For this review, take the finished solid that the model builds, in its own axes (mm). A direction names the side the tool comes from. Coordinates: 2 decimals unless noted, no trailing zeros. Loops run counter-clockwise (first coordinate to the right, second up) from the corner with the lowest first, then second, coordinate; pieces in that order, holes last.
1. Take a section at C-C, the plane x = -23. State the section outline as (y, z) points, then the cut area to 3 significant figures.
2. Machinability: for faces 4 (the face through (11, 4, -27)), 5 (the face through (8.8, 6, -13)), 6 (the face through (-37.564, 3.944, -30.454)), 7 (the face through (-26, 4, 22.486)), which of the approach directions +Z, -Z, +X, -X, +Y, -Y give a long, thin tool a straight path to every point of the face, cutting with its end or side? Answer none if there is none.
3. Clearance check with flat-ended pins moving along their axes: P1, Ø1.5, axis at y = 4, z = 2.5, coming from the +X side; P2, Ø5.5, axis at x = -10.61, z = 10.61, coming from the +Y side; P3, Ø1.8, axis at x = -10.5, z = 24.5, coming from the -Y side. State where each tip first meets the part, or that it passes through.
4. Take a section at D-D, the plane z = 3.5. State the section outline as (x, y) points.
5. To check wall thickness, follow probe 1 along Z at (x, y) = (-30, 1); probe 2 along X at (y, z) = (5.5, 12.5); probe 3 along X at (y, z) = (6, 12). State the ranges of each line that lie inside material, in increasing order.
6. Mouldability with a two-part tool opening along X and no side actions: class faces 1 (the face through (3, 4, 32.014)), 2 (the face through (-37.53, 3.94, 30.6)), 3 (the face through (8.899, 5.972, -27.372)) as pulls with the +X half, pulls with the -X half, needs draft (parallel to the pull), parting line crosses it, or undercut.
7. Take a section at A-A, the plane x = 0. State the section outline as (y, z) points, then the cut area to 3 significant figures.
8. Take a section at B-B, the plane z = -26. State the section outline as (x, y) points.
```python
from build123d import *

# Parameters (mm, degrees)
SKETCH1_R           = 9
SKETCH1_R_2         = 1.5
SKETCH1_W           = 17.49
SKETCH1_H           = 7
SKETCH1_W_2         = 18.51
BOSS_EXTRUDE1_DEPTH = 8
SKETCH2_R           = 3
CUT_EXTRUDE1_DEPTH  = 4
SKETCH5_R           = 1.5
CUT_EXTRUDE3_DEPTH  = 52.125968688
SKETCH5_3_R         = 3
SKETCH5_3_R_2       = 1.5
CUT_EXTRUDE4_DEPTH  = 4


with BuildPart() as part:
    # Sketch1 → Boss-Extrude1 (new body)
    with BuildSketch(Plane(origin=(0, 0, 0), x_dir=(1, 0, 0), z_dir=(0, 1, 0))):
        with BuildLine():
            Line((-33.922517503, 31.986083161), (38.983038853, 31.986083161))
            Line((38.983038853, 31.986083161), (39.05091296, -32.013916839))
            Line((39.05091296, -32.013916839), (-34.065012631, -32.013916839))
            ThreePointArc((-34.065012631, -32.013916839), (-37.566569007, -30.563524698), (-39.016961147, -27.061968322))
            Line((-39.016961147, -27.061968322), (-39.016961147, 26.891639518))
            ThreePointArc((-39.016961147, 26.891639518), (-37.52483315, 30.493955165), (-33.922517503, 31.986083161))
        make_face()
        with Locations(Location((0, 0, 0), (0, 0, 270))):
            Circle(SKETCH1_R, mode=Mode.SUBTRACT)
        with Locations(Location((10.606601718, 10.606601718, 0), (0, 0, 270))):
            Circle(SKETCH1_R_2, mode=Mode.SUBTRACT)
        with Locations(Location((-10.606601718, 10.606601718, 0), (0, 0, 90))):
            Circle(SKETCH1_R_2, mode=Mode.SUBTRACT)
        with Locations(Location((10.606601718, -10.606601718, 0), (0, 0, 90))):
            Circle(SKETCH1_R_2, mode=Mode.SUBTRACT)
        with Locations(Location((-10.606601718, -10.606601718, 0), (0, 0, 270))):
            Circle(SKETCH1_R_2, mode=Mode.SUBTRACT)
        with Locations((-26.271961147, 25.986083161)):
            Rectangle(SKETCH1_W, SKETCH1_H, mode=Mode.SUBTRACT)
        with Locations((26.728038853, 25.986083161)):
            Rectangle(SKETCH1_W_2, SKETCH1_H, mode=Mode.SUBTRACT)
        with Locations((26.728038853, -25.986083161)):
            Rectangle(SKETCH1_W_2, SKETCH1_H, mode=Mode.SUBTRACT)
        with Locations((-26.271961147, -25.986083161)):
            Rectangle(SKETCH1_W, SKETCH1_H, mode=Mode.SUBTRACT)
    extrude(amount=BOSS_EXTRUDE1_DEPTH)

    # Sketch2 → Cut-Extrude1 (cut)
    with BuildSketch(Plane(origin=(0, 8, 0), x_dir=(1, 0, 0), z_dir=(0, 1, 0))):
        with Locations(Location((10.606601718, 10.606601718, 0), (0, 0, 270))):
            Circle(SKETCH2_R)
        with Locations(Location((10.606601718, -10.606601718, 0), (0, 0, 270))):
            Circle(SKETCH2_R)
        with Locations(Location((-10.606601718, -10.606601718, 0), (0, 0, 270))):
            Circle(SKETCH2_R)
        with Locations(Location((-10.606601718, 10.606601718, 0), (0, 0, 270))):
            Circle(SKETCH2_R)
    extrude(amount=-CUT_EXTRUDE1_DEPTH, mode=Mode.SUBTRACT)

    # Sketch5 → Cut-Extrude3 (cut, through all)
    with BuildSketch(Plane.XZ):
        with Locations(Location((-10.52309756, 25.986083161, 0), (0, 0, 270))):
            Circle(SKETCH5_R)
        with Locations(Location((9.473038853, 25.986083161, 0), (0, 0, 270))):
            Circle(SKETCH5_R)
        with Locations(Location((9.473038853, -25.986083161, 0), (0, 0, 270))):
            Circle(SKETCH5_R)
        with Locations(Location((-10.52309756, -25.986083161, 0), (0, 0, 270))):
            Circle(SKETCH5_R)
    extrude(amount=-CUT_EXTRUDE3_DEPTH, mode=Mode.SUBTRACT)

    # Sketch5_3 → Cut-Extrude4 (cut)
    # profile 1 of 4: a face of its own
    with BuildSketch(Plane.XZ):
        with Locations(Location((-10.52309756, -25.986083161, 0), (0, 0, 270))):
            Circle(SKETCH5_3_R)
        with Locations(Location((-10.52309756, -25.986083161, 0), (0, 0, 270))):
            Circle(SKETCH5_3_R_2, mode=Mode.SUBTRACT)
    # profile 2 of 4: a face of its own
    with BuildSketch(Plane.XZ):
        with Locations(Location((9.473038853, -25.986083161, 0), (0, 0, 270))):
            Circle(SKETCH5_3_R)
        with Locations(Location((9.473038853, -25.986083161, 0), (0, 0, 270))):
            Circle(SKETCH5_3_R_2, mode=Mode.SUBTRACT)
    # profile 3 of 4: a face of its own
    with BuildSketch(Plane.XZ):
        with Locations(Location((9.473038853, 25.986083161, 0), (0, 0, 270))):
            Circle(SKETCH5_3_R)
        with Locations(Location((9.473038853, 25.986083161, 0), (0, 0, 270))):
            Circle(SKETCH5_3_R_2, mode=Mode.SUBTRACT)
    # profile 4 of 4: a face of its own
    with BuildSketch(Plane.XZ):
        with Locations(Location((-10.52309756, 25.986083161, 0), (0, 0, 270))):
            Circle(SKETCH5_3_R)
        with Locations(Location((-10.52309756, 25.986083161, 0), (0, 0, 270))):
            Circle(SKETCH5_3_R_2, mode=Mode.SUBTRACT)
    extrude(amount=-CUT_EXTRUDE4_DEPTH, mode=Mode.SUBTRACT)


solid = part.part
```
Results list:
1. outline: (0, -31.99) - (8, -31.99) - (8, -29.49) - (0, -29.49) - close; (0, -22.49) - (8, -22.49) - (8, 22.49) - (0, 22.49) - close; (0, 29.49) - (8, 29.49) - (8, 32.01) - (0, 32.01) - close
1. area: 400 mm2
2. face 4: -Y
2. face 5: +Y
2. face 6: -Z, -X, +Y, -Y
2. face 7: +Y, -Y
3. P1: stops at x = 39.02
3. P2: stops at y = 4
3. P3: stops at y = 4
4. outline: (-39.02, 0) - (-8.29, 0) - (-8.29, 8) - (-39.02, 8) - close; (8.29, 0) - (39.02, 0) - (39.02, 8) - (8.29, 8) - close
5. probe 1: z = -31.99 to -29.49, -22.49 to 22.49, 29.49 to 32.01
5. probe 2: x = -39.02 to -12.93, -8.28 to 8.28, 12.93 to 39.03
5. probe 3: x = -39.02 to -13.26, -7.95 to 7.95, 13.26 to 39.03
6. face 1: needs draft
6. face 2: pulls with the -X half
6. face 3: undercut
7. outline: (0, -31.99) - (8, -31.99) - (8, -9) - (0, -9) - close; (0, 9) - (8, 9) - (8, 32.01) - (0, 32.01) - close
7. area: 368 mm2
8. outline: (-39.02, 0) - (-35.02, 0) - (-35.02, 8) - (-39.02, 8) - close; (-17.53, 0) - (-13.52, 0) - (-13.52, 4) - (-12.02, 4) - (-12.02, 8) - (-17.53, 8) - close; (-9.02, 4) - (-7.52, 4) - (-7.52, 0) - (6.47, 0) - (6.47, 4) - (7.97, 4) - (7.97, 8) - (-9.02, 8) - close; (10.97, 4) - (12.47, 4) - (12.47, 0) - (17.47, 0) - (17.47, 8) - (10.97, 8) - close; (35.98, 0) - (38.99, 0) - (38.99, 8) - (35.98, 8) - close
